Geometry: final body of the model. Coordinates: model frame, mm. A direction names the side the tool comes from. Give positions to 0.01 mm unless a question says otherwise; leave off trailing zeros. Loops run counter-clockwise (first coordinate to the right, second up) from the corner with the lowest first, then second, coordinate; pieces in that order, holes last. Notation, with made-up numbers: (37, 16.5) - (65, 16.5) arc R15 ccw to (65, 36.5) - close; hole circle Ø10 at (-5.75, 78). An arc over 180 degrees is marked (long way). Use one line per item in the form item = value.
```python
from build123d import *

# Parameters (mm, degrees)
BOX_W           = 25
BOX_H           = 14
BOX_DEPTH       = 35
SKETCH_W        = 25
SKETCH_H        = 3.4
POCKET_DEPTH    = 25
SKETCH001_R     = 2.45
POCKET001_DEPTH = 8
SKETCH002_R     = 1.4
POCKET002_DEPTH = 6.001
SKETCH003_W     = 4
SKETCH003_H     = 4
PAD_DEPTH       = 4
CHAMFER_SIZE    = 1.99
POCKET003_DEPTH = 17
CHAMFER001_SIZE = 8
CHAMFER002_SIZE = 6
CHAMFER003_SIZE = 6
CHAMFER004_SIZE = 1.5
CHAMFER005_SIZE = 1.4
CHAMFER006_SIZE = 1.2
CHAMFER007_SIZE = 1.5


with BuildPart() as pocket002:
    # Box → Box (new body)
    with BuildSketch(Plane.XY):
        with Locations((12.5, 7)):
            Rectangle(BOX_W, BOX_H)
    extrude(amount=BOX_DEPTH)

    # Sketch → Pocket (cut)
    with BuildSketch(Plane.XY.offset(35)):
        with Locations((12.5, 3.7)):
            Rectangle(SKETCH_W, SKETCH_H)
    extrude(amount=-POCKET_DEPTH, mode=Mode.SUBTRACT)

    # Sketch001 → Pocket001 (cut)
    with BuildSketch(Plane.XZ):
        with Locations((18.55, 6.45)):
            Circle(SKETCH001_R)
    extrude(amount=-POCKET001_DEPTH, mode=Mode.SUBTRACT)

    # Sketch002 → Pocket002 (cut, through all)
    with BuildSketch(Plane.XZ.offset(-8)):
        with Locations((18.55, 6.45)):
            Circle(SKETCH002_R)
    extrude(amount=-POCKET002_DEPTH, mode=Mode.SUBTRACT)


with BuildPart() as chamfer007:
    # Sketch003 → Pad (new body)
    with BuildSketch(Plane.XZ):
        with Locations((12.5, 25)):
            Rectangle(SKETCH003_W, SKETCH003_H)
    extrude(amount=-PAD_DEPTH)

    # Chamfer
    chamfer_edges = [chamfer007.edges().sort_by_distance(p)[0] for p in [
        (12.5, 4, 23),
        (10.5, 4, 25),
        (12.5, 4, 27),
        (14.5, 4, 25),
    ]]
    chamfer(chamfer_edges, length=CHAMFER_SIZE)

    # Fusion: union Pocket002
    add(pocket002.part)

    # Sketch005 → Pocket003 (cut)
    with BuildSketch(Plane.XZ):
        with BuildLine():
            ThreePointArc((19.539949, 7.439949), (17.560051, 7.439949), (17.560051, 5.460051))
            Line((17.560051, 5.460051), (0, 23.020101))
            Line((0, 26.979899), (0, 23.020101))
            Line((19.539949, 7.439949), (0, 26.979899))
        make_face()
    extrude(amount=-POCKET003_DEPTH, mode=Mode.SUBTRACT)

    # Chamfer001
    chamfer001_edges = [chamfer007.edges().sort_by_distance(p)[0] for p in [
        (0, 7, 0),
    ]]
    chamfer(chamfer001_edges, length=CHAMFER001_SIZE)

    # Chamfer002
    chamfer002_edges = [chamfer007.edges().sort_by_distance(p)[0] for p in [
        (25, 7, 0),
    ]]
    chamfer(chamfer002_edges, length=CHAMFER002_SIZE)

    # Chamfer003
    chamfer003_edges = [chamfer007.edges().sort_by_distance(p)[0] for p in [
        (0, 9.7, 35),
        (25, 9.7, 35),
        (0, 1, 35),
        (25, 1, 35),
        (12.5, 14, 35),
    ]]
    chamfer(chamfer003_edges, length=CHAMFER003_SIZE)

    # Chamfer004
    chamfer004_edges = [chamfer007.edges().sort_by_distance(p)[0] for p in [
        (20.12237, 0, 8.32887),
    ]]
    chamfer(chamfer004_edges, length=CHAMFER004_SIZE)

    # Chamfer005
    chamfer005_edges = [chamfer007.edges().sort_by_distance(p)[0] for p in [
        (19.085757, 14, 5.156569),
    ]]
    chamfer(chamfer005_edges, length=CHAMFER005_SIZE)

    # Chamfer006
    chamfer006_edges = [chamfer007.edges().sort_by_distance(p)[0] for p in [
        (12.5, 2, 35),
    ]]
    chamfer(chamfer006_edges, length=CHAMFER006_SIZE)

    # Chamfer007
    chamfer007_edges = [chamfer007.edges().sort_by_distance(p)[0] for p in [
        (12.5, 5.4, 35),
    ]]
    chamfer(chamfer007_edges, length=CHAMFER007_SIZE)


solid = chamfer007.part
```
(1) Access query for faces 1 (the face through (9.92, 13.31, 18.06)), 2 (the face through (8.9, 7.61, 14.12)), 3 (the face through (22, 7, 3)), 4 (the face through (23, 9, 31)), 5 (the face through (4, 5.4, 14)). Directions: +Z, -Z, +X, -X, +Y, -Y. A direction counts if a zero-diameter tool reaches every point of the face in a straight line with its end or side. Return the directions, or none.
Solution:
face_1 = +Y
face_2 = +Y, -Y
face_3 = -Z, +X, +Y, -Y
face_4 = +Z, +X, +Y, -Y
face_5 = +Z, +X, -X
(2) Cut plane D-D (x = 10). Return the cut outline in (y, z), plus the area to 3 significant figures.
Solution:
outline = (0, 0) - (14, 0) - (14, 11.04) - (12.6, 13.02) - (5.4, 13.02) - (5.4, 10) - (2, 10) - (2, 13.02) - (0, 13.02) - close; (0, 16.98) - (2, 16.98) - (2, 33.8) - (0.8, 35) - (0, 35) - close; (5.4, 16.98) - (12.6, 16.98) - (14, 18.96) - (14, 29) - (8, 35) - (6.9, 35) - (5.4, 33.5) - close
area = 340 mm2
(3) Cut plane A-A (y = 3.5). Return the cut outline in (x, z), plus the area to 3 significant figures.
Solution:
outline = (0, 8) - (8, 0) - (19, 0) - (25, 6) - (25, 10) - (16.98, 10) - (18.12, 8.86) arc R2.45 cw (long way) to (16.14, 6.88) - (13.02, 10) - (0, 10) - close; (11.99, 24.49) - (13.01, 24.49) - (13.01, 25.51) - (11.99, 25.51) - close
area = 175 mm2
(4) Cut plane B-B (x = 18.55). Return the cut outline in (y, z).
Solution:
outline = (0, 0) - (14, 0) - (14, 3.65) - (12.6, 5.05) - (8, 5.05) - (8, 4) - (1.5, 4) - (0, 2.5) - close; (0, 10.4) - (1.5, 8.9) - (8, 8.9) - (8, 8.43) - (12.6, 8.43) - (14, 10.41) - (14, 29) - (8, 35) - (6.9, 35) - (5.4, 33.5) - (5.4, 10) - (2, 10) - (2, 33.8) - (0.8, 35) - (0, 35) - close
(5) Cut plane C-C (z = 28.5). Return the cut outline in (x, y), plus the area to 3 significant figures.
Solution:
outline = (0, 0) - (25, 0) - (25, 2) - (0, 2) - close; (0, 5.4) - (25, 5.4) - (25, 14) - (0.46, 14) - (0, 13.67) - close
area = 265 mm2
(6) Material intervals for L1, parallel to Y at x = 2.5, z = 14; L2, parallel to X at y = 5, z = 6.45; L3, parallel to Z at x = 18.55, y = 6.75, sorted ascending. Write a range as from..to.
Solution:
L1 = 0..2, 5.4..14
L2 = 1.55..16.1, 21..25
L3 = 0..4, 8.9..34.85
(7) Pull-direction query (Y, two-part tool) for faces 6 (the face through (0, 1, 28)), 7 (the face through (20, 8, 5)), 8 (the face through (15, 5.4, 25)); classes: released by +Y, released by -Y, zero draft, split by the parting line, or undercut.
Solution:
face_6 = zero draft
face_7 = released by -Y
face_8 = undercut
(8) Pin query (flat end, axial travel): P1, Ø2.5, axis at x = 21, y = 4, coming from the +Z side; P2, Ø3, axis at x = 18.55, z = 6.45, coming from the -Y side; P3, Ø5.5, axis at x = 18, z = 7, coming from the -Y side. Return the tip coordinate at first contact, or that it passes through.
Solution:
P1 = 10
P2 = 8
P3 = 0.51
